```python
from build123d import *

# Parameters (mm, degrees)
SKETCH_13_R                      = 2.6
SM_BASE_FLANGE_2_DEPTH           = 4
SM_EDGE_FLANGE_2_STRIP_W         = 24
SM_EDGE_FLANGE_2_STRIP_H         = 4
SM_EDGE_FLANGE_2_STRIP_CUT_DEPTH = 120
SM_EDGE_FLANGE_2_DEPTH           = 120
FILLET_1_R                       = 5
FILLET_2_R                       = 3
FILLET_3_R                       = 10
SKETCH_23_R                      = 2.6
CUT_EXTRUDE_2_DEPTH              = 10


# Sheet-metal steps are written as plain solids
with BuildPart() as part:
    # Эскиз13 → Базовая кромка2 (new body)
    with BuildSketch(Plane.XY):
        with BuildLine():
            Line((-60, 0), (60, 0))
            Line((60, 0), (60, 12))
            Line((60, 12), (50, 12))
            Line((50, 12), (20, 126.23475383))
            ThreePointArc((20, 126.23475383), (0, 130), (-20, 126.23475383))
            Line((-20, 126.23475383), (-50, 12))
            Line((-50, 12), (-60, 12))
            Line((-60, 12), (-60, 0))
        make_face()
        with Locations((0, 75)):
            Circle(SKETCH_13_R, mode=Mode.SUBTRACT)
        with BuildLine():
            ThreePointArc((9.731596096, 111.318811068), (0, 112.6), (-9.731596096, 111.318811068))
            ThreePointArc((-9.731596096, 111.318811068), (-11.570073727, 108.134474403), (-8.385737061, 106.295996772))
            ThreePointArc((-8.385737061, 106.295996772), (0, 107.4), (8.385737061, 106.295996772))
            ThreePointArc((8.385737061, 106.295996772), (11.570073727, 108.134474403), (9.731596096, 111.318811068))
        make_face(mode=Mode.SUBTRACT)
        with BuildLine():
            ThreePointArc((-9.731596096, 38.681188932), (0, 37.4), (9.731596096, 38.681188932))
            ThreePointArc((9.731596096, 38.681188932), (11.570073727, 41.865525597), (8.385737061, 43.704003228))
            ThreePointArc((8.385737061, 43.704003228), (0, 42.6), (-8.385737061, 43.704003228))
            ThreePointArc((-8.385737061, 43.704003228), (-11.570073727, 41.865525597), (-9.731596096, 38.681188932))
        make_face(mode=Mode.SUBTRACT)
    extrude(amount=-SM_BASE_FLANGE_2_DEPTH)

    # Ребро-кромка2 strip (across the edge) → Ребро-кромка2 strip cut (cut)
    with BuildSketch(Plane.YZ.offset(-60)):
        with Locations((-4, -2)):
            Rectangle(SM_EDGE_FLANGE_2_STRIP_W, SM_EDGE_FLANGE_2_STRIP_H)
    extrude(amount=SM_EDGE_FLANGE_2_STRIP_CUT_DEPTH, mode=Mode.SUBTRACT)

    # Ребро-кромка2 section (across the edge) → Ребро-кромка2 (add)
    with BuildSketch(Plane.YZ.offset(-60)):
        with BuildLine():
            Line((0, 4), (0, 36))
            Line((0, 36), (4, 36))
            Line((4, 36), (4, 4))
            ThreePointArc((4, 4), (5.171572875, 1.171572875), (8, 0))
            Line((8, 0), (8, -4))
            ThreePointArc((8, -4), (2.343145751, -1.656854249), (0, 4))
        make_face()
    extrude(amount=SM_EDGE_FLANGE_2_DEPTH)

    # Скругление1
    fillet_1_edges = [part.edges().sort_by_distance(p)[0] for p in [
        (-50, 12, -2),
        (50, 12, -2),
    ]]
    fillet(fillet_1_edges, radius=FILLET_1_R)

    # Скругление2
    fillet_2_edges = [part.edges().sort_by_distance(p)[0] for p in [
        (-60, 12, -2),
        (-20, 126.23475383, -2),
        (20, 126.23475383, -2),
        (60, 12, -2),
    ]]
    fillet(fillet_2_edges, radius=FILLET_2_R)

    # Скругление3
    fillet_3_edges = [part.edges().sort_by_distance(p)[0] for p in [
        (-60, 2, 36),
        (60, 2, 36),
    ]]
    fillet(fillet_3_edges, radius=FILLET_3_R)

    # Эскиз23 → Вырез-Вытянуть2 (cut)
    with BuildSketch(Plane(origin=(0, 4, 0), x_dir=(1, 0, 0), z_dir=(0, 1, 0))):
        with Locations(Location((-50, -26, 0), (0, 0, 270))):
            Circle(SKETCH_23_R)
        with Locations(Location((50, -26, 0), (0, 0, 270))):
            Circle(SKETCH_23_R)
        with Locations(Location((0, -10, 0), (0, 0, 270))):
            Circle(SKETCH_23_R)
    extrude(amount=-CUT_EXTRUDE_2_DEPTH, mode=Mode.SUBTRACT)


solid = part.part
```
Work out the finished part from the listing and answer in its coordinate system (mm). A direction names the side the tool comes from. Round coordinates to 2 decimals unless told otherwise and drop trailing zeros. Write each loop counter-clockwise with the first axis right and the second up, starting at its lowest first coordinate (ties: lowest second). Pieces come first, ordered by that corner, then holes.
1) A cutting plane is placed at B-B on z = 10. Determine the outline of the cut face in (x, y), and give its area (3 significant figures).
2) Flat-ended cylindrical pins translate along their axes: P1, Ø1.5, axis at x = -41, z = 26.5, coming from the -Y side; P2, Ø8.5, axis at x = -50, z = 26, coming from the +Y side; P3, Ø2.5, axis at x = 55.5, z = -1.5, coming from the +Y side; P4, Ø3, axis at x = 0, y = 75, coming from the -Z side. Find the tip coordinate at first contact, or state that the pin passes through.
3) A cutting plane is placed at D-D on z = 21. Determine the outline of the cut face in (x, y), and give its area (3 significant figures).
4) Determine the mould class of faces 4 (the face through (-1, 56, -4)), 5 (the face through (11.584, 41.81, -1.972)), 6 (the face through (34.9, 69.5, -2)) for opening direction Y: pulls with the +Y half, pulls with the -Y half, needs draft (parallel to the pull), parting line crosses it, or undercut.
5) A cutting plane is placed at C-C on y = 75. Determine the outline of the cut face in (x, z).
6) Consider probe 1 along X at (y, z) = (2.7, 26); probe 2 along X at (y, z) = (2, 10); probe 3 along Y at (x, z) = (46.5, 33). Determine where each line is inside the solid, lowest interval first.
7) A cutting plane is placed at A-A on x = 0. Determine the outline of the cut face in (y, z), and give its area (4 significant figures).
8) Which of the six approach directions +Z, -Z, +X, -X, +Y, -Y give full straight-line access (tool end or side, diameter ignored) to faces 1 (the face through (-1, 4, 20)), 2 (the face through (0.1, 42.6, -2)), 3 (the face through (0, 130, -2))?
Entries:
1. outline: (-60, 0) - (-2.6, 0) - (-2.6, 4) - (-60, 4) - close; (2.6, 0) - (60, 0) - (60, 4) - (2.6, 4) - close
1. area: 459 mm2
2. P1: stops at y = 0
2. P2: stops at y = 4
2. P3: stops at y = 12
2. P4: passes through
3. outline: (-60, 0) - (60, 0) - (60, 4) - (-60, 4) - close
3. area: 480 mm2
4. face 4: needs draft
4. face 5: undercut
4. face 6: pulls with the +Y half
5. outline: (-33.46, -4) - (-2.6, -4) - (-2.6, 0) - (-33.46, 0) - close; (2.6, -4) - (33.46, -4) - (33.46, 0) - (2.6, 0) - close
6. probe 1: x = -60 to -52.6, -47.4 to 47.4, 52.6 to 60
6. probe 2: x = -60 to -2.6, 2.6 to 60
6. probe 3: y = 0 to 4
7. outline: (0, 4) arc R8 ccw to (8, -4) - (37.4, -4) - (37.4, 0) - (8, 0) arc R4 cw to (4, 4) - (4, 7.4) - (0, 7.4) - close; (0, 12.6) - (4, 12.6) - (4, 36) - (0, 36) - close; (42.6, -4) - (72.4, -4) - (72.4, 0) - (42.6, 0) - close; (77.6, -4) - (107.4, -4) - (107.4, 0) - (77.6, 0) - close; (112.6, -4) - (130, -4) - (130, 0) - (112.6, 0) - close
7. area: 570.5 mm2
8. face 1: +Z, +X, -X, +Y
8. face 2: +Z, -Z
8. face 3: +Z, -Z, +Y
